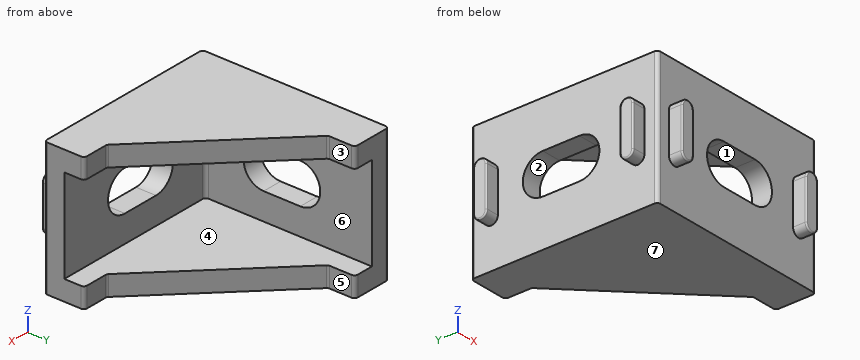
```python
from build123d import *

# Parameters (mm, degrees)
BOSS_EXTRUDE1_DEPTH = 20
SKETCH2_W           = 25
SKETCH2_H           = 14
CUT_EXTRUDE1_DEPTH  = 25
CUT_EXTRUDE2_DEPTH  = 29
BOSS_EXTRUDE2_DEPTH = 2
FILLET4_R           = 0.5
FILLET5_R           = 0.2


with BuildPart() as part:
    # Sketch1 → Boss-Extrude1 (new body)
    with BuildSketch(Plane.XY):
        Polygon((-8, 10), (-8, 14), (-14, 14), (-14, -14), (14, -14), (14, -8), (10, -8), align=None)
    extrude(amount=BOSS_EXTRUDE1_DEPTH)

    # Sketch2 → Cut-Extrude1 (cut)
    with BuildSketch(Plane(origin=(0, 14, 0), x_dir=(1, 0, 0), z_dir=(0, 1, 0))):
        with Locations((1.5, -10)):
            Rectangle(SKETCH2_W, SKETCH2_H)
    extrude(amount=-CUT_EXTRUDE1_DEPTH, mode=Mode.SUBTRACT)

    # Sketch3 → Cut-Extrude2 (cut, through all)
    with BuildSketch(Plane.XZ.offset(14)):
        with BuildLine():
            Line((-2.25, 13), (3.25, 13))
            ThreePointArc((3.25, 13), (6.25, 10), (3.25, 7))
            Line((3.25, 7), (-2.25, 7))
            ThreePointArc((-2.25, 7), (-5.25, 10), (-2.25, 13))
        make_face()
    cut_extrude2 = extrude(amount=-CUT_EXTRUDE2_DEPTH, mode=Mode.SUBTRACT)

    # Mirror1: Cut-Extrude2 across plane
    add(cut_extrude2.mirror(Plane(origin=(0, 0, 0), x_dir=(0, 0, 1), z_dir=(-0.707106781, 0.707106781, 0))), mode=Mode.SUBTRACT)

    # Sketch4 → Boss-Extrude2 (add)
    with BuildSketch(Plane.ZY.offset(14)):
        with BuildLine():
            Line((7, 12), (13, 12))
            ThreePointArc((13, 12), (14, 11), (13, 10))
            Line((13, 10), (7, 10))
            ThreePointArc((7, 10), (6, 11), (7, 12))
        make_face()
        with BuildLine():
            Line((7, -12), (13, -12))
            ThreePointArc((13, -12), (14, -11), (13, -10))
            Line((13, -10), (7, -10))
            ThreePointArc((7, -10), (6, -11), (7, -12))
        make_face()
    boss_extrude2 = extrude(amount=BOSS_EXTRUDE2_DEPTH)

    # Mirror4: Boss-Extrude2 across plane
    add(boss_extrude2.mirror(Plane(origin=(0, 0, 0), x_dir=(0, 0, 1), z_dir=(-0.707106781, 0.707106781, 0))))

    # Fillet4
    fillet4_edges = [part.edges().sort_by_distance(p)[0] for p in [
        (14, -8, 18.5),
        (14, -14, 10),
        (-14, -14, 10),
        (-14, 14, 10),
        (-8, 14, 18.5),
        (-8, 10, 18.5),
        (10, -8, 18.5),
        (14, -8, 1.5),
        (-8, 14, 1.5),
        (-8, 10, 1.5),
        (10, -8, 1.5),
        (-11, -11, 10),
    ]]
    fillet(fillet4_edges, radius=FILLET4_R)

    # Fillet5
    fillet5_edges = [part.edges().sort_by_distance(p)[0] for p in [
        (-16, -11, 6),
        (-16, -12, 10),
        (-16, -11, 14),
        (-16, -10, 10),
        (11, -16, 6),
        (12, -16, 10),
        (11, -16, 14),
        (10, -16, 10),
        (-11, -16, 6),
        (-10, -16, 10),
        (-11, -16, 14),
        (-12, -16, 10),
        (-16, 11, 6),
        (-16, 10, 10),
        (-16, 11, 14),
        (-16, 12, 10),
    ]]
    fillet(fillet5_edges, radius=FILLET5_R)


solid = part.part
```
Could you check a few things on this model? Use its own coordinates, in mm. Face numbers are marked on the shaded views. A direction names the side the tool comes from. Coordinates: 2 decimals unless noted, no trailing zeros. Write each loop counter-clockwise with the first axis right and the second up, starting at its lowest first coordinate (ties: lowest second). Pieces come first, ordered by that corner, then holes. Notation, with made-up numbers: (54.25, -23.5) - (83.25, -23.5) arc R19 ccw to (83.25, 5.5) - close; hole circle Ø5 at (8, 76). An arc over 180 degrees is marked (long way). Use a Markdown table: item, result.
Q1. Thinking about a two-plate mould opening in Z: for the marked faces 4, 5, 6 and 7, which applies, +Z half, -Z half, draft (parallel to the pull), parting line (faces both ways), or undercut?
Geometry check:
| item | result |
|---|---|
| face 4 | undercut |
| face 5 | draft |
| face 6 | undercut |
| face 7 | -Z half |
Q2. Imagine slicing it at A-A (x = -5.75). List the corners of the cut face in (y, z) for me.
Geometry check:
| item | result |
|---|---|
| outline | (-14, 0) - (7.75, 0) - (7.75, 3) - (-11, 3) - (-11, 17) - (7.75, 17) - (7.75, 20) - (-14, 20) - close |
Q3. Imagine slicing it at D-D (x = 7). List the corners of the cut face in (y, z) for me.
Geometry check:
| item | result |
|---|---|
| outline | (-14, 0) - (-5, 0) - (-5, 3) - (-11, 3) - (-11, 17) - (-5, 17) - (-5, 20) - (-14, 20) - close |
Q4. Imagine slicing it at B-B (z = 18.5). List the corners of the cut face in (x, y) for me.
Geometry check:
| item | result |
|---|---|
| outline | (-14, -13.5) arc R0.5 ccw to (-13.5, -14) - (13.5, -14) arc R0.5 ccw to (14, -13.5) - (14, -8.5) arc R0.5 ccw to (13.5, -8) - (10.21, -8) arc R0.5 cw to (9.85, -7.85) - (-7.85, 9.85) arc R0.5 cw to (-8, 10.21) - (-8, 13.5) arc R0.5 ccw to (-8.5, 14) - (-13.5, 14) arc R0.5 ccw to (-14, 13.5) - close |
Q5. I'm going to push flat-ended pins straight in: pin 1 Ø2 at (x, z) = (-4, 7.5) entering from -Y; pin 2 Ø0.9 at (y, z) = (-15, 11.5) entering from +X; pin 3 Ø6 at (x, z) = (5.5, 16.5) entering from +Y; pin 4 Ø5 at (x, y) = (-1.5, 7.5) entering from +Z. Where does each tip first touch, or does it pass through?
Geometry check:
| item | result |
|---|---|
| pin 1 | stops at y = -14 |
| pin 2 | stops at x = 12 |
| pin 3 | stops at y = -0.54 |
| pin 4 | passes through |
Q6. Please list where these lines run through material, in increasing order: L1, parallel to Z at x = -8.5, y = 8; L2, parallel to Y at x = -12.5, z = 10; L3, parallel to Z at x = 1.5, y = -11.5.
Geometry check:
| item | result |
|---|---|
| L1 | z = 0 to 3, 17 to 20 |
| L2 | y = -14 to -5.25, 6.25 to 14 |
| L3 | z = 0 to 7, 13 to 20 |
Q7. Imagine slicing it at C-C (y = 11). List the corners of the cut face in (x, z) for me, and give its area (3 significant figures).
Geometry check:
| item | result |
|---|---|
| outline | (-16, 6.2) arc R0.2 ccw to (-15.8, 6) - (-14, 6) - (-14, 0) - (-8, 0) - (-8, 3) - (-11, 3) - (-11, 17) - (-8, 17) - (-8, 20) - (-14, 20) - (-14, 14) - (-15.8, 14) arc R0.2 ccw to (-16, 13.8) - close |
| area | 94.0 mm2 |
Q8. Which directions (+Z, -Z, +X, -X, +Y, -Y) give clear straight access to the entire face, cutting with the end or side of a thin tool? Please do the marked faces 1, 2 and 3.
Geometry check:
| item | result |
|---|---|
| face 1 | +Y, -Y |
| face 2 | +X, -X |
| face 3 | +Z, -Z, +X, +Y |
